from build123d import *

# Parameters (mm, degrees)
SKETCH1_W                                            = 38.00356671
SKETCH1_H                                            = 25.735371596
SKETCH1_R                                            = 1.5
SKETCH1_R_2                                          = 2.5
BOSS_EXTRUDE1_DEPTH                                  = 3.175
SKETCH2_W                                            = 38.00356671
SKETCH2_H                                            = 3.342685798
BOSS_EXTRUDE2_DEPTH                                  = 16
SKETCH3_R                                            = 5
SKETCH3_R_2                                          = 2
CUT_EXTRUDE1_DEPTH                                   = 10
ESCAREADO_PARA_PARAFUSO_DE_M_QUINA_COM_C_D           = 4
ESCAREADO_PARA_PARAFUSO_DE_M_QUINA_COM_C_CSINK_D     = 9.4
ESCAREADO_PARA_PARAFUSO_DE_M_QUINA_COM_C_CSINK_ANGLE = 90


with BuildPart() as part:
    # Sketch1 → Boss-Extrude1 (new body)
    with BuildSketch(Plane.XY):
        Rectangle(SKETCH1_W, SKETCH1_H)
        with Locations((-14.5, -1.307314202)):
            Circle(SKETCH1_R, mode=Mode.SUBTRACT)
        with Locations((14.5, -1.307314202)):
            Circle(SKETCH1_R, mode=Mode.SUBTRACT)
        with Locations((0, -1.307314202)):
            Circle(SKETCH1_R_2, mode=Mode.SUBTRACT)
        with Locations((0, -9.132314202)):
            Circle(SKETCH1_R, mode=Mode.SUBTRACT)
    extrude(amount=BOSS_EXTRUDE1_DEPTH)

    # Sketch2 → Boss-Extrude2 (add)
    with BuildSketch(Plane(origin=(0, 0, 0), x_dir=(-1, 0, 0), z_dir=(0, 0, -1))):
        with Locations((0, 11.196342899)):
            Rectangle(SKETCH2_W, SKETCH2_H)
    extrude(amount=BOSS_EXTRUDE2_DEPTH)

    # Sketch3 → Cut-Extrude1 (cut)
    with BuildSketch(Plane.XZ.offset(-9.525)):
        with Locations((4.5, -9.5)):
            Circle(SKETCH3_R)
        with Locations((-14, -9.5)):
            Circle(SKETCH3_R_2)
        with Locations((14, -9.5)):
            Circle(SKETCH3_R_2)
    extrude(amount=-CUT_EXTRUDE1_DEPTH, mode=Mode.SUBTRACT)

    # Escareado para parafuso de máquina com cabeça chata de M42 (through all)
    with Locations(Plane(origin=(0, 12.867685798, 0), x_dir=(-1, 0, 0), z_dir=(0, 1, 0))):
        with Locations((14, -9.5), (-14, -9.5)):
            CounterSinkHole(ESCAREADO_PARA_PARAFUSO_DE_M_QUINA_COM_C_D / 2, ESCAREADO_PARA_PARAFUSO_DE_M_QUINA_COM_C_CSINK_D / 2, counter_sink_angle=ESCAREADO_PARA_PARAFUSO_DE_M_QUINA_COM_C_CSINK_ANGLE)


solid = part.part
Build history of the part. All positions in model axes, mm. A direction names the side the tool comes from. Coordinates: 2 decimals unless noted, no trailing zeros. Order: outer loops, then holes, each group sorted by start corner. A loop starts at its lowest first (then second) coordinate and runs counter-clockwise, first axis right, second up. Notation, with made-up numbers: (26, 43) -> (60, 43) arc R11 ccw to (60, 48) -> close; hole circle Ø8 at (72, 67). An arc over 180 degrees is marked (long way). One line per item, written item: value.
(1) Probe line 1 (X direction, y = 9.7, z = -9.5); line 2 (Y direction, x = 0, z = 1.6); line 3 (X direction, y = 11, z = -9.5). List the from-to ranges inside material, lowest first. Write a range as [from, to].
Checked values:
line 1: [-19, -16], [-12, -0.5], [9.5, 12], [16, 19]
line 2: [-12.87, -10.63], [-7.63, -3.81], [1.19, 12.87]
line 3: [-19, -16.83], [-11.17, -0.5], [9.5, 11.17], [16.83, 19]
(2) Tool access for faces 1 (the cylindrical face through (1.344, 0.801, 1.565)), 2 (the flat face through (0, 9.525, -6)): list every direction of +Z, -Z, +X, -X, +Y, -Y with a clear straight run to the whole face (end or side of a thin tool).
Checked values:
face 1: +Z, -Z
face 2: -Z, +X, -X, -Y
(3) Slice it at D-D, the plane x = 0. List the corners of the cut face in (y, z) (3 decimals), plus the area to 3 significant figures.
Checked values:
outline: (-12.868, 0) -> (-10.632, 0) -> (-10.632, 3.175) -> (-12.868, 3.175) -> close; (-7.632, 0) -> (-3.807, 0) -> (-3.807, 3.175) -> (-7.632, 3.175) -> close; (1.193, 0) -> (9.525, 0) -> (9.525, -7.321) -> (12.868, -7.321) -> (12.868, 3.175) -> (1.193, 3.175) -> close; (9.525, -16) -> (12.868, -16) -> (12.868, -11.679) -> (9.525, -11.679) -> close
area: 95.2 mm2
(4) Drop flat-ended pins along their axis: pin 1 Ø1 at (x, z) = (-13.5, -4) entering from -Y (3 decimals); pin 2 Ø6.5 at (x, z) = (14, -9.5) entering from +Y; pin 3 Ø4 at (x, y) = (0, -9.13) entering from -Z. Give the stop position or say it passes through.
Checked values:
pin 1: y = 9.525
pin 2: y = 11.42
pin 3: z = 0
(5) Slice it at B-B, the plane x = -14. List the corners of the cut face in (y, z) (3 decimals).
Checked values:
outline: (-12.868, 0) -> (-2.722, 0) -> (-2.722, 3.175) -> (-12.868, 3.175) -> close; (0.107, 0) -> (9.525, 0) -> (9.525, -7.5) -> (10.168, -7.5) -> (12.868, -4.8) -> (12.868, 3.175) -> (0.107, 3.175) -> close; (9.525, -16) -> (12.868, -16) -> (12.868, -14.2) -> (10.168, -11.5) -> (9.525, -11.5) -> close
(6) Slice it at C-C, the plane z = 1.25. List the corners of the cut face in (x, y).
Checked values:
outline: (-19, -12.87) -> (19, -12.87) -> (19, 12.87) -> (-19, 12.87) -> close; hole circle Ø3 at (-14.5, -1.31); hole circle Ø5 at (0, -1.31); hole circle Ø3 at (0, -9.13); hole circle Ø3 at (14.5, -1.31)
(7) Slice it at A-A, the plane x = 4.5. List the corners of the cut face in (y, z) (3 decimals).
Checked values:
outline: (-12.868, 0) -> (9.525, 0) -> (9.525, -4.5) -> (12.868, -4.5) -> (12.868, 3.175) -> (-12.868, 3.175) -> close; (9.525, -16) -> (12.868, -16) -> (12.868, -14.5) -> (9.525, -14.5) -> close
(8) Mould opens along X. For faces 3 (the cylindrical face through (-0.495, 11.173, -9.28)), 4 (the flat face through (19.002, 2, 1)), 5 (the flat face through (0, -4, 0)) say: pulls with the +X half, pulls with the -X half, needs draft (parallel to the pull), parting line crosses it, or undercut.
Checked values:
face 3: undercut
face 4: pulls with the +X half
face 5: needs draft
